Part model, mm, in its own coordinate system. A direction names the side the tool comes from. Coordinates: 2 decimals unless noted, no trailing zeros. Loops run counter-clockwise (first coordinate to the right, second up) from the corner with the lowest first, then second, coordinate; pieces in that order, holes last.
Autodesk Inventor part; units mm, degrees
ref_plane "MSC_PF1" through (0, 0, 0) normal (1, 0, 0) x (0, 1, 0)
ref_plane "MSC_PT1" through (0, 0, 0) normal (0, 0, -1) x (-1, 0, 0)
ref_plane "YZ Plane" through (0, 0, 0) normal (1, 0, 0) x (0, 1, 0)
sketch "Szkic1" plane through (0, 0, 0) normal (0, 1, 0) x (-1, 0, 0)
  point P0 (0, 0)
sketch "Szkic2" plane through (0, 0, 0) normal (0, 1, 0) x (-1, 0, 0)
  line L0 (-2.5, -16) -> (0, -16)
  line L1 (-2.5, -2.8) -> (-2.5, -16)
  line L2 (-5, -0.3) -> (-2.5, -2.8)
  line L3 (-5, 0) -> (-5, -0.3)
  line L4 (0, 0) -> (-5, 0)
  line L5 (0, -16) -> (0, 0)
  line L6 (0, -16) -> (0, 0)
  line L7 (0, -19.2) -> (0, 3.2)
  line L8 (1, 0) -> (-6, 0)
  dimension "d3" = 5
  dimension "d5" = 2.5
  dimension "d7" = 16
  dimension "ParC" = 0.3
  dimension "d22" = 0
  dimension "d23" = 0
  dimension "d43" = 45
revolve "Obrót1" add sketch "Szkic2" angle 360 about axis through (0, 0, -16) along (0, 0, -1)
sketch "Szkic3" plane through (0, 0, 0) normal (0, 0, 1) x (1, 0, 0)
  line L0 (-1.5, 0.866) -> (-1.5, -0.866)
  line L1 (0, 1.7321) -> (-1.5, 0.866)
  line L2 (1.5, 0.866) -> (0, 1.7321)
  line L3 (1.5, -0.866) -> (1.5, 0.866)
  line L4 (0, -1.7321) -> (1.5, -0.866)
  line L5 (-1.5, -0.866) -> (0, -1.7321)
  circle A0 centre (0, 0) radius 1.5 construction
  circle A1 centre (0, 0) radius 2.5 construction
  dimension "d11" = 3
  dimension "d13" = 120
  dimension "d15" = 120
extrude "Wyciągnięcie proste1" cut sketch "Szkic3" against normal blind 2.3
fillet "Zaokrąglenie1" radius 0.2 1 edges at (-2.5, 0, -2.8)
chamfer "Faza1" distance 0.4 angle 45 1 edges at (-2.5, 0, -16) measured on face at (-0.599, -2.4272, -11.6276)
thread "Gwint1"
ref_plane "MSC_PF1" through (0, 0, 0) normal (1, 0, 0) x (0, 1, 0)
ref_plane "MSC_PT1" through (0, 0, 0) normal (0, 0, -1) x (-1, 0, 0)
equation "\"d3\" = 0.5 * dk"
equation "\"d5\" = 0.5 * NND"
equation "\"d7\" = NLG"
equation "\"d43\" = 0.5 * ang"
equation "\"d11\" = ParS"
equation "\"d16\" = ParT"
equation "\"d18\" = r"
equation "\"d19\" = 0.5 * PTC"
equation "\"d39\" = 0.5 * PTC"
equation "\"NND\" = 5"
equation "\"PTC\" = 0.8"
equation "\"ParK\" = 2.8"
equation "\"ParS\" = 3"
equation "\"ParT\" = 2.3"
equation "\"r\" = 0.2"
equation "\"NLG\" = 16"
equation "\"ang\" = 90deg"
equation "\"THREADDIA\" = NND"
properties part number "DIN 7991 - M5x16" material "Stal, miękka"
Q1. Saw through at A-A (z = -1). List the corners of the cut face in (x, y).
Q2. Probe line 1 (Y direction, x = 0, z = -12.75); line 2 (Y direction, x = -2, z = -13.25); line 3 (Z direction, x = -0.25, y = 1). List the from-to ranges inside material, lowest first.
Q3. Mould opens along Y. For faces 4 (the flat face through (2, 0, 0)), 5 (the flat face through (0.74, -1.305, -1.134)), 6 (the flat face through (0.76, 1.293, -1.134)), 7 (the conical face through (2.586, 0.814, -2.589)) say: released by +Y, released by -Y, zero draft, split by the parting line, or undercut.
Q4. Tool access for faces 1 (the flat face through (1.5, 0, -1)), 2 (the cylindrical face through (4.77, -1.5, -0.15)), 3 (the cylindrical face through (-0.54, 2.44, -9.33)): list every direction of +Z, -Z, +X, -X, +Y, -Y with a clear straight run to the whole face (end or side of a thin tool).
Q5. Drop flat-ended pins along their axis: P1, Ø1.9, axis at y = 0, z = -1.5, coming from the +X side; P2, Ø1, axis at y = -2.5, z = -8.5, coming from the +X side; P3, Ø0.5, axis at y = 0, z = -1.5, coming from the -X side. Give the stop position or say it passes through.
Q6. Saw through at B-B (z = -10.75). List the corners of the cut face in (x, y), plus the area to 3 significant figures.
Checked values:
1. outline: circle Ø8.6 at (0, 0); hole (-1.5, -0.87) - (0, -1.73) - (1.5, -0.87) - (1.5, 0.87) - (0, 1.73) - (-1.5, 0.87) - close
2. line 1: y = -2.5 to 2.5
2. line 2: y = -1.5 to 1.5
2. line 3: z = -16 to -2.3
3. face 4: zero draft
3. face 5: undercut
3. face 6: undercut
3. face 7: split by the parting line
4. face 1: +Z
4. face 2: +Z, -Z
4. face 3: -Z
5. P1: stops at x = 4.75
5. P2: stops at x = 1.5
5. P3: stops at x = -4.05
6. outline: circle Ø5 at (0, 0)
6. area: 19.6 mm2
